from build123d import *

# Parameters (mm, degrees)
SKETCH_1_W      = 165
SKETCH_1_H      = 100
EXTRUDE_1_DEPTH = 5
SKETCH_2_R      = 1.65
SKETCH_2_W      = 165
SKETCH_2_H      = 1.53
SKETCH_2_H_2    = 4.42
SKETCH_2_H_3    = 100
EXTRUDE_2_DEPTH = 1.65


with BuildPart() as part:
    # 草图1 → 凸台-拉伸1 (new body)
    with BuildSketch(Plane(origin=(0, 0, 0), x_dir=(1, 0, 0), z_dir=(0, 1, 0))):
        with Locations((8.779069767, 0)):
            Rectangle(SKETCH_1_W, SKETCH_1_H)
    extrude(amount=EXTRUDE_1_DEPTH)

    # 草图2 → 凸台-拉伸2 (add)
    # profile 1 of 7: a face of its own
    with BuildSketch(Plane.XZ):
        with BuildLine():
            Line((83.279069767, 51.53), (91.279069767, 51.53))
            Line((91.279069767, 51.53), (91.279069767, 56.63))
            ThreePointArc((91.279069767, 56.63), (90.136786214, 59.387716447), (87.379069767, 60.53))
            Line((87.379069767, 60.53), (87.179069767, 60.53))
            ThreePointArc((87.179069767, 60.53), (84.421353321, 59.387716447), (83.279069767, 56.63))
            Line((83.279069767, 56.63), (83.279069767, 51.53))
        make_face()
        with Locations(Location((87.279069767, 56.63, 0), (0, 0, 270))):
            Circle(SKETCH_2_R, mode=Mode.SUBTRACT)
    # profile 2 of 7: a face of its own
    with BuildSketch(Plane.XZ):
        with Locations((8.779069767, 50.765)):
            Rectangle(SKETCH_2_W, SKETCH_2_H)
    # profile 3 of 7: a face of its own
    with BuildSketch(Plane.XZ):
        with BuildLine():
            Line((-73.720930233, 56.63), (-73.720930233, 51.53))
            Line((-73.720930233, 51.53), (-65.720930233, 51.53))
            Line((-65.720930233, 51.53), (-65.720930233, 56.63))
            ThreePointArc((-65.720930233, 56.63), (-66.863213786, 59.387716447), (-69.620930233, 60.53))
            Line((-69.620930233, 60.53), (-69.820930233, 60.53))
            ThreePointArc((-69.820930233, 60.53), (-72.578646679, 59.387716447), (-73.720930233, 56.63))
        make_face()
        with Locations(Location((-69.720930233, 56.63, 0), (0, 0, 270))):
            Circle(SKETCH_2_R, mode=Mode.SUBTRACT)
    # profile 4 of 7: a face of its own
    with BuildSketch(Plane.XZ):
        with BuildLine():
            Line((-65.720930233, -54.42), (-73.720930233, -54.42))
            Line((-73.720930233, -54.42), (-73.720930233, -59.52))
            ThreePointArc((-73.720930233, -59.52), (-72.578646679, -62.277716447), (-69.820930233, -63.42))
            Line((-69.820930233, -63.42), (-69.620930233, -63.42))
            ThreePointArc((-69.620930233, -63.42), (-66.863213786, -62.277716447), (-65.720930233, -59.52))
            Line((-65.720930233, -59.52), (-65.720930233, -54.42))
        make_face()
        with Locations(Location((-69.720930233, -59.52, 0), (0, 0, 270))):
            Circle(SKETCH_2_R, mode=Mode.SUBTRACT)
    # profile 5 of 7: a face of its own
    with BuildSketch(Plane.XZ):
        with Locations((8.779069767, -52.21)):
            Rectangle(SKETCH_2_W, SKETCH_2_H_2)
    # profile 6 of 7: a face of its own
    with BuildSketch(Plane.XZ):
        with BuildLine():
            Line((91.279069767, -59.52), (91.279069767, -54.42))
            Line((91.279069767, -54.42), (83.279069767, -54.42))
            Line((83.279069767, -54.42), (83.279069767, -59.52))
            ThreePointArc((83.279069767, -59.52), (84.421353321, -62.277716447), (87.179069767, -63.42))
            Line((87.179069767, -63.42), (87.379069767, -63.42))
            ThreePointArc((87.379069767, -63.42), (90.136786214, -62.277716447), (91.279069767, -59.52))
        make_face()
        with Locations(Location((87.279069767, -59.52, 0), (0, 0, 270))):
            Circle(SKETCH_2_R, mode=Mode.SUBTRACT)
    # profile 7 of 7: a face of its own
    with BuildSketch(Plane.XZ):
        with Locations((8.779069767, 0)):
            Rectangle(SKETCH_2_W, SKETCH_2_H_3)
    extrude(amount=EXTRUDE_2_DEPTH)


solid = part.part
Geometry: final body of the model. Coordinates: model frame, mm. A direction names the side the tool comes from. Coordinates: 2 decimals unless noted, no trailing zeros. Loops run counter-clockwise (first coordinate to the right, second up) from the corner with the lowest first, then second, coordinate; pieces in that order, holes last. Notation, with made-up numbers: (40.25, 7) - (96.25, 7) arc R14 ccw to (96.25, 26) - close; hole circle Ø11 at (8.5, 61.5). An arc over 180 degrees is marked (long way). One line per question, with ' | ' between items. Start each with the question number.
(1) Cut plane A-A on x = -56. Output: boundary loops of the cut face in (y, z).
(2) Ray query, L1, parallel to X at y = -1, z = 56.63; L2, parallel to Z at x = -22, y = 1.5; L3, parallel to Z at x = 26, y = -0.25. Return the intervals inside material, ascending. Write a range as from..to.
(3) Reachability of faces 1 (the cylindrical face through (84.452, -0.813, 59.418)), 2 (the flat face through (8, 0, -52)), 3 (the cylindrical face through (84.391, -0.813, -62.247)), 4 (the flat face through (8, 2, 50)), 5 (the cylindrical face through (87.35, -0.81, 58.28)) from +Z, -Z, +X, -X, +Y, -Y: full face, straight path, thin tool, end or side. Return the list, or none.
(4) Cut plane B-B on y = 3.25. Output: boundary loops of the cut face in (x, z).
(5) Draft query along Z for faces 6 (the flat face through (91.279, 2, -2)), 7 (the cylindrical face through (-72.548, -0.813, 59.418)), 8 (the cylindrical face through (88.67, -0.81, -60.41)), 9 (the cylindrical face through (-69.225, -0.813, -61.094)). Return one class per face: +Z half, -Z half, draft (parallel to the pull), parting line (faces both ways), or undercut.
(6) First-contact query: pin 1 (5.5 mm diameter, centred on x = 87.28, z = -59.52, fed in from +Y); pin 2 (2 mm diameter, centred on x = -69.72, z = 56.63, fed in from +Y); pin 3 (1.5 mm diameter, centred on x = 0, y = 2, fed in from -Z); pin 4 (1.3 mm diameter, centred on x = -10.5, y = -0.5, fed in from +Z). Flat tips, straight axial feed; report the tip coordinate or a pass-through.
Here are the results:
1) outline: (-1.65, -54.42) - (0, -54.42) - (0, -50) - (5, -50) - (5, 50) - (0, 50) - (0, 51.53) - (-1.65, 51.53) - close
2) L1: -73.72..-71.37, -68.07..-65.72, 83.28..85.63, 88.93..91.28 | L2: -50..50 | L3: -54.42..51.53
3) face 1: +Z, +Y, -Y | face 2: -Z, +X, -X, +Y | face 3: -Z, +Y, -Y | face 4: +Z, +X, -X, +Y | face 5: +Y, -Y
4) outline: (-73.72, -50) - (91.28, -50) - (91.28, 50) - (-73.72, 50) - close
5) face 6: draft | face 7: +Z half | face 8: undercut | face 9: undercut
6) pin 1: y = 0 | pin 2: through | pin 3: z = -50 | pin 4: z = 51.53
